```python
from build123d import *

# Parameters (mm, degrees)
SKETCH_1_R      = 1.6
EXTRUDE_1_DEPTH = 3
FILLET_1_R      = 3


with BuildPart() as part:
    # 草图1 → 凸台-拉伸1 (new body)
    with BuildSketch(Plane.XY):
        Polygon((8, 11), (-8, 11), (-23, -6), (-31, -6), (-31, 4), (-7.5, 30.633333333), (-7.5, 41), (7.5, 41), (7.5, 30.633333333), (31, 4), (31, -6), (23, -6), align=None)
        with Locations((-25, 0)):
            Circle(SKETCH_1_R, mode=Mode.SUBTRACT)
        with Locations((25, 0)):
            Circle(SKETCH_1_R, mode=Mode.SUBTRACT)
        with Locations((0, 35)):
            Circle(SKETCH_1_R, mode=Mode.SUBTRACT)
        with Locations((0, 15)):
            Circle(SKETCH_1_R, mode=Mode.SUBTRACT)
    extrude(amount=EXTRUDE_1_DEPTH)

    # 圆角1
    fillet_1_edges = [part.edges().sort_by_distance(p)[0] for p in [
        (23, -6, 1.5),
        (8, 11, 1.5),
        (-8, 11, 1.5),
        (-23, -6, 1.5),
        (-31, -6, 1.5),
        (-31, 4, 1.5),
        (-7.5, 30.633333333, 1.5),
        (-7.5, 41, 1.5),
        (7.5, 41, 1.5),
        (7.5, 30.633333333, 1.5),
        (31, 4, 1.5),
        (31, -6, 1.5),
    ]]
    fillet(fillet_1_edges, radius=FILLET_1_R)


solid = part.part
```
Read the model definition and answer for the solid it produces. Units are mm, in the model's axes. A direction names the side the tool comes from. Give positions to 0.01 mm unless a question says otherwise; leave off trailing zeros. Order: outer loops, then holes, each group sorted by start corner. A loop starts at its lowest first (then second) coordinate and runs counter-clockwise, first axis right, second up. Notation, with made-up numbers: (37, -15.75) -> (52, -15.75) arc R27 ccw to (52, 1.25) -> close; hole circle Ø6 at (-26.5, 3). An arc over 180 degrees is marked (long way). One line per item, written item: value. Start each with the question number.
(1) A tool of negligible diameter and unlimited length cuts with its end or side. For faces 4 (the flat face through (7.5, 35, 1)), 5 (the flat face through (26, -6, 1)), 6 (the flat face through (31, 0, 1)), 7 (the flat face through (15.59, 2.4, 1.48)), 8 (the flat face through (-7.5, 35, 1)), from which of +Z, -Z, +X, -X, +Y, -Y can it reach the whole face along a straight path? Write none if from no direction.
(2) The part is cut by section B-B (y = 35). Determine the outline of the cut face in (x, z), and give its area (3 significant figures).
(3) The part is cut by section A-A (x = 25). Determine the outline of the cut face in (y, z).
(4) The part is cut by section C-C (x = 0). Determine the outline of the cut face in (y, z).
(5) The part is cut by section D-D (z = 1.65). Determine the outline of the cut face in (x, y), and give its area (3 significant figures).
(6) For a pull along X with two mould halves and no side action, classify faces 1 (the cylindrical face through (23.104, -5.727, 1.521)), 2 (the cylindrical face through (30.811, 3.912, 1.521)), 3 (the cylindrical face through (-6.64, 40.1, 1.52)) as released by +X, released by -X, zero draft, split by the parting line, or undercut.
(7) Flat-ended cylindrical pins translate along their axes: P1, Ø1.5, axis at x = 2, z = 1, coming from the -Y side; P2, Ø1.5, axis at y = 19, z = 2, coming from the -X side. Find the tip coordinate at first contact, or state that the pin passes through.
(8) Straight lines are drawn through the part: L1, parallel to Y at x = 0, z = 0.8; L2, parallel to X at y = -1, z = 1.5; L3, parallel to Y at x = -1, z = 1.35. For each, find the intervals that lie inside material, in ascending order.
Taken from the geometry:
1. face 4: +Z, -Z, +X, +Y
1. face 5: +Z, -Z, +X, -X, -Y
1. face 6: +Z, -Z, +X, +Y, -Y
1. face 7: +Z, -Z, -Y
1. face 8: +Z, -Z, -X, +Y
2. outline: (-7.5, 0) -> (-1.6, 0) -> (-1.6, 3) -> (-7.5, 3) -> close; (1.6, 0) -> (7.5, 0) -> (7.5, 3) -> (1.6, 3) -> close
2. area: 35.4 mm^2
3. outline: (-6, 0) -> (-1.6, 0) -> (-1.6, 3) -> (-6, 3) -> close; (1.6, 0) -> (10.8, 0) -> (10.8, 3) -> (1.6, 3) -> close
4. outline: (11, 0) -> (13.4, 0) -> (13.4, 3) -> (11, 3) -> close; (16.6, 0) -> (33.4, 0) -> (33.4, 3) -> (16.6, 3) -> close; (36.6, 0) -> (41, 0) -> (41, 3) -> (36.6, 3) -> close
5. outline: (-31, -3) arc R3 ccw to (-28, -6) -> (-24.35, -6) arc R3 ccw to (-22.1, -4.98) -> (-8.9, 9.98) arc R3 cw to (-6.65, 11) -> (6.65, 11) arc R3 cw to (8.9, 9.98) -> (22.1, -4.98) arc R3 ccw to (24.35, -6) -> (28, -6) arc R3 ccw to (31, -3) -> (31, 2.87) arc R3 ccw to (30.25, 4.85) -> (8.25, 29.78) arc R3 cw to (7.5, 31.77) -> (7.5, 38) arc R3 ccw to (4.5, 41) -> (-4.5, 41) arc R3 ccw to (-7.5, 38) -> (-7.5, 31.77) arc R3 cw to (-8.25, 29.78) -> (-30.25, 4.85) arc R3 ccw to (-31, 2.87) -> close; hole circle Ø3.2 at (-25, 0); hole circle Ø3.2 at (0, 15); hole circle Ø3.2 at (0, 35); hole circle Ø3.2 at (25, 0)
5. area: 1,230 mm^2
6. face 1: undercut
6. face 2: released by +X
6. face 3: released by -X
7. P1: y = 11
7. P2: x = -18.43
8. L1: 11 to 13.4, 16.6 to 33.4, 36.6 to 41
8. L2: -31 to -26.25, -23.75 to -18.59, 18.59 to 23.75, 26.25 to 31
8. L3: 11 to 13.75, 16.25 to 33.75, 36.25 to 41
